Geometry: final body of the model. Coordinates: model frame, mm. A direction names the side the tool comes from. Give positions to 0.01 mm unless a question says otherwise; leave off trailing zeros. Order: outer loops, then holes, each group sorted by start corner. A loop starts at its lowest first (then second) coordinate and runs counter-clockwise, first axis right, second up. Notation, with made-up numbers: (-1, 38.25) -> (57, 38.25) arc R29 cw to (57, 68.25) -> close; hole circle Ø11 at (22.5, -35). An arc over 180 degrees is marked (long way). Answer in a Markdown table with one row per item. Add a question column.
Q1. Cut plane B-B on z = -28. Return the cut outline in (x, y).
Q2. Line query: line 1 along X through (y, z) = (8.5, -40); line 2 along X through (y, z) = (3.5, -78.5); line 3 along Y through (x, z) = (330, -15). Output: solid intervals per line, ascending. Write a range as from..to.
Q3. Cut plane A-A on y = 13. Return the cut outline in (x, z).
Q4. Set-up query: faces 1 (the face through (44, 19, -38.1)), 2 (the face through (0, 19, -63)), 3 (the face through (407.988, 9, -45)), 4 (the face through (819, 19, -50.8)). Return all of +Z, -Z, +X, -X, +Y, -Y with unobstructed straight access to the full face (end or side cutting, diameter ignored); none if empty.
Q5. Contact query for flat-ended pins moving along their axis: P1, Ø19, axis at y = 19, z = -14, coming from the -X side; P2, Ø6, axis at x = 397.5, z = -58, coming from the -Y side; P3, Ø19, axis at y = 22.5, z = -77, coming from the +X side. Output: stop coordinate, or through.
Q6. Cut plane C-C on x = 798.5. Return the cut outline in (y, z).
Q7. Pull-direction query (X, two-part tool) for faces 5 (the face through (319.088, 9, -45)), 6 (the face through (471, 19, 0)), 7 (the face through (863.6, 19, -25)), 8 (the face through (363, 19.05, -44)); classes: +X half, -X half, draft (parallel to the pull), parting line (faces both ways), or undercut.
from build123d import *

# Parameters (mm, degrees)
SKETCH1_W           = 863.6
SKETCH1_H           = 88.9
BOSS_EXTRUDE1_DEPTH = 38.1
SKETCH2_W           = 88.9
SKETCH2_H           = 88.9
CUT_EXTRUDE1_DEPTH  = 19.05
SKETCH3_W           = 88.9
SKETCH3_H           = 38.1
CUT_EXTRUDE2_DEPTH  = 39.1
SKETCH4_W           = 88.9
SKETCH4_H           = 38.1
CUT_EXTRUDE3_DEPTH  = 39.1


with BuildPart() as part:
    # Sketch1 → Boss-Extrude1 (new body)
    with BuildSketch(Plane(origin=(0, 0, 0), x_dir=(1, 0, 0), z_dir=(0, 1, 0))):
        with Locations((431.8, 44.45)):
            Rectangle(SKETCH1_W, SKETCH1_H)
    extrude(amount=BOSS_EXTRUDE1_DEPTH)

    # Sketch2 → Cut-Extrude1 (cut)
    with BuildSketch(Plane.XZ):
        with Locations((363.5375, -44.45)):
            Rectangle(SKETCH2_W, SKETCH2_H)
    extrude(amount=-CUT_EXTRUDE1_DEPTH, mode=Mode.SUBTRACT)

    # Sketch3 → Cut-Extrude2 (cut, through all)
    with BuildSketch(Plane(origin=(0, 38.1, 0), x_dir=(1, 0, 0), z_dir=(0, 1, 0))):
        with Locations((44.45, 19.05)):
            Rectangle(SKETCH3_W, SKETCH3_H)
    extrude(amount=-CUT_EXTRUDE2_DEPTH, mode=Mode.SUBTRACT)

    # Sketch4 → Cut-Extrude3 (cut, through all)
    with BuildSketch(Plane(origin=(0, 38.1, 0), x_dir=(1, 0, 0), z_dir=(0, 1, 0))):
        with Locations((819.15, 69.85)):
            Rectangle(SKETCH4_W, SKETCH4_H)
    extrude(amount=-CUT_EXTRUDE3_DEPTH, mode=Mode.SUBTRACT)


solid = part.part
Completed:
| question | item | result |
|---|---|---|
| 1 | outline | (88.9, 0) -> (319.09, 0) -> (319.09, 19.05) -> (407.99, 19.05) -> (407.99, 0) -> (863.6, 0) -> (863.6, 38.1) -> (88.9, 38.1) -> close |
| 2 | line 1 | x = 0..319.09, 407.99..863.6 |
| 2 | line 2 | x = 0..319.09, 407.99..774.7 |
| 2 | line 3 | y = 19.05..38.1 |
| 3 | outline | (0, -88.9) -> (319.09, -88.9) -> (319.09, 0) -> (88.9, 0) -> (88.9, -38.1) -> (0, -38.1) -> close; (407.99, -88.9) -> (774.7, -88.9) -> (774.7, -50.8) -> (863.6, -50.8) -> (863.6, 0) -> (407.99, 0) -> close |
| 4 | face 1 | +Z, -X, +Y, -Y |
| 4 | face 2 | +Z, -Z, -X, +Y, -Y |
| 4 | face 3 | +Z, -Z, -Y |
| 4 | face 4 | -Z, +X, +Y, -Y |
| 5 | P1 | stops at x = 88.9 |
| 5 | P2 | stops at y = 19.05 |
| 5 | P3 | stops at x = 774.7 |
| 6 | outline | (0, -50.8) -> (38.1, -50.8) -> (38.1, 0) -> (0, 0) -> close |
| 7 | face 5 | undercut |
| 7 | face 6 | draft |
| 7 | face 7 | +X half |
| 7 | face 8 | undercut |
